Autodesk Inventor part; units mm, degrees
ref_plane "YZ Plane" through (0, 0, 0) normal (1, 0, 0) x (0, 1, 0)
ref_plane "XZ Plane" through (0, 0, 0) normal (0, 1, 0) x (-1, 0, 0)
ref_plane "XY Plane" through (0, 0, 0) normal (0, 0, 1) x (1, 0, 0)
sketch "Sketch1" plane through (0, 0, 0) normal (0, 0, 1) x (1, 0, 0)
  line L0 (-5.4972, 0.152) -> (-2.6169, 4.8367)
  line L1 (-2.6169, 4.8367) -> (2.8802, 4.6847)
  line L2 (2.8802, 4.6847) -> (5.4972, -0.152)
  line L3 (5.4972, -0.152) -> (2.6169, -4.8367)
  line L4 (2.6169, -4.8367) -> (-2.8802, -4.6847)
  line L5 (-2.8802, -4.6847) -> (-5.4972, 0.152)
  circle A0 centre (0, 0) radius 12.7
  dimension "d0" = 9.525
  dimension "d1" = 25.4
extrude "Extrusion1" add sketch "Sketch1" along normal blind 77.47
sketch "Sketch3" plane through (0, 0, 77.47) normal (0, 0, 1) x (1, 0, 0)
  line L0 (-5.4972, 0.152) -> (-2.6169, 4.8367)
  line L1 (-5.4972, 0.152) -> (-2.6169, 4.8367)
  line L2 (-2.6169, 4.8367) -> (2.8802, 4.6847)
  line L3 (2.8802, 4.6847) -> (5.4972, -0.152)
  line L4 (5.4972, -0.152) -> (2.6169, -4.8367)
  line L5 (2.6169, -4.8367) -> (-2.8802, -4.6847)
  line L6 (-2.8802, -4.6847) -> (-5.4972, 0.152)
  circle A0 centre (0, 0) radius 19.05
  dimension "d4" = 38.1
extrude "Extrusion2" add sketch "Sketch3" along normal blind 3.175
sketch "Sketch4" plane through (0, 0, 0) normal (0, 0, -1) x (-1, 0, 0)
  line L0 (-5.4972, -0.152) -> (-2.8802, 4.6847)
  line L1 (-2.8802, 4.6847) -> (2.6169, 4.8367)
  line L2 (2.6169, 4.8367) -> (5.4972, 0.152)
  line L3 (5.4972, 0.152) -> (2.8802, -4.6847)
  line L4 (2.8802, -4.6847) -> (-2.6169, -4.8367)
  line L5 (-2.6169, -4.8367) -> (-5.4972, -0.152)
  line L6 (2.8802, -4.6847) -> (-2.6169, -4.8367)
  circle A0 centre (0, 0) radius 19.05
  dimension "d7" = 9.525
  dimension "d8" = 180
  dimension "d11" = 38.1
extrude "Extrusion3" add sketch "Sketch4" along normal blind 3.175
properties part number "Polycord conveyor"
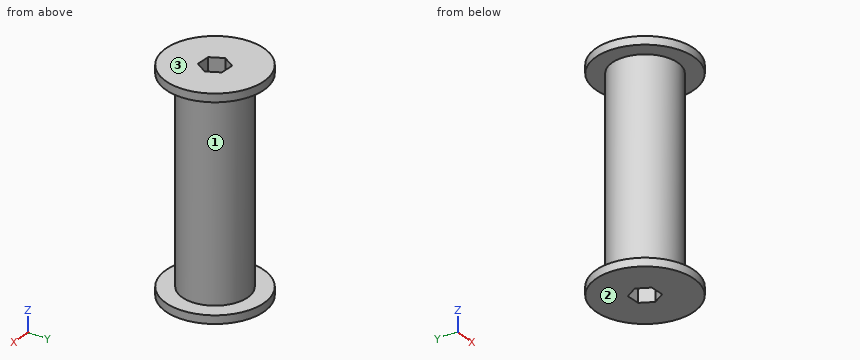
The model under review builds one solid part; all positions refer to its coordinate system, in mm. Face numbers are marked on the shaded views. Give positions to 0.01 mm unless a question says otherwise; leave off trailing zeros. Order: outer loops, then holes, each group sorted by start corner. A loop starts at its lowest first (then second) coordinate and runs counter-clockwise, first axis right, second up. Notation, with made-up numbers: M 87,-2.5 L 140,-2.5 A24 cw 140,27.5 Z; hole C 36,19 d3. An arc over 180 degrees is marked long. Use one line per item in the form item = value. Start each with the question number.
Item 1: We need section C-C on z = 9.5. Give the boundary of the cut face in (x, y), plus the area to 3 significant figures.
Item 2: The part is to be moulded in two halves that separate along Z. For the marked faces 1, 2 and 3, say which applies: pulls with the +Z half, pulls with the -Z half, needs draft (parallel to the pull), parting line crosses it, or undercut.
Item 3: We need section B-B on y = -3. Give the boundary of the cut face in (x, z) (3 decimals).
Item 4: To check wall thickness, follow line 1 along Z through (x, y) = (-0.5, -15.5) (3 decimals); line 2 along X through (y, z) = (-2, 55); line 3 along Y through (x, z) = (2.5, 73). State the ranges of each line that lie inside material, in increasing order. Write a range as from..to.
Item 5: We need section A-A on x = 0. Give the boundary of the cut face in (y, z) (3 decimals), plus the area to 3 significant figures.
Item 6: Insertion check: pin 1 Ø12 at (x, z) = (3, 22) entering from -Y; pin 2 Ø4 at (y, z) = (7.5, 14) entering from -X; pin 3 Ø2 at (y, z) = (-7, 10.5) entering from -X. Each pin has a flat end and moves straight along its axis. Give the tip position at first contact, or say it passes through.
Item 7: We need section D-D on x = 13.5. Give the boundary of the cut face in (y, z) (3 decimals).
Completed:
q1.outline = C 0,0 d25.4; hole M -5.5,0.15 L -2.88,-4.68 L 2.62,-4.84 L 5.5,-0.15 L 2.88,4.68 L -2.62,4.84 Z
q1.area = 428 mm²
q2.face_1 = undercut
q2.face_2 = pulls with the -Z half
q2.face_3 = pulls with the +Z half
q3.outline = M -18.812,-3.175 L -3.792,-3.175 L -3.792,80.645 L -18.812,80.645 L -18.812,77.47 L -12.341,77.47 L -12.341,0 L -18.812,0 Z; M 3.746,-3.175 L 18.812,-3.175 L 18.812,0 L 12.341,0 L 12.341,77.47 L 18.812,77.47 L 18.812,80.645 L 3.746,80.645 Z
q4.line_1 = -3.175..0, 77.47..80.645
q4.line_2 = -12.54..-4.33, 4.36..12.54
q4.line_3 = -12.45..-4.83, 4.7..12.45
q5.outline = M -19.05,-3.175 L -4.764,-3.175 L -4.764,80.645 L -19.05,80.645 L -19.05,77.47 L -12.7,77.47 L -12.7,0 L -19.05,0 Z; M 4.764,-3.175 L 19.05,-3.175 L 19.05,0 L 12.7,0 L 12.7,77.47 L 19.05,77.47 L 19.05,80.645 L 4.764,80.645 Z
q5.area = 1,410 mm²
q6.pin_1 = -12.7
q6.pin_2 = -11.45
q6.pin_3 = -11.19
q7.outline = M -13.441,-3.175 L 13.441,-3.175 L 13.441,0 L -13.441,0 Z; M -13.441,77.47 L 13.441,77.47 L 13.441,80.645 L -13.441,80.645 Z
